Could you check a few things on this drawing? It's one solid part, dimensions in mm from its lowest x, y, z. A direction names the side the tool comes from. Coordinates: 2 decimals unless noted, no trailing zeros. Loops run counter-clockwise (first coordinate to the right, second up) from the corner with the lowest first, then second, coordinate; pieces in that order, holes last. Notation, with made-up numbers: M -22.5,4.5 L 30.5,4.5 A13 ccw 30.5,18.5 Z; hole C 30,74.25 d11. An arc over 180 degrees is marked long. Answer as a JSON object with one key per item and string values. Group by question number.
Item 1: Which directions (+Z, -Z, +X, -X, +Y, -Y) give clear straight access to the entire face, cutting with the end or side of a thin tool? Please do the marked faces 1 and 2.
Item 2: Suppose I cut it at B-B (y = 38.1). Write out the boundary of the cut face in (x, z) (1 decimal).
Item 3: If I drill on line 1 (Y direction, x = 18, z = 38) (1 decimal); line 2 (X direction, y = 38, z = 23); line 3 (X direction, y = 38.1, z = 26.5), over which ranges is the centre line in solid material (lowest first)?
Item 4: I'm going to push flat-ended pins straight in: pin 1 Ø3 at (y, z) = (18, 38) entering from +X; pin 2 Ø1.5 at (x, z) = (58.5, 33.5) entering from -Y. Where does each tip first touch, or does it pass through?
Item 5: We'd pull the mould along Y, two halves only. Please class the marked faces 3, 4, 5 and 6: +Y half, -Y half, draft (parallel to the pull), parting line (faces both ways), or undercut.
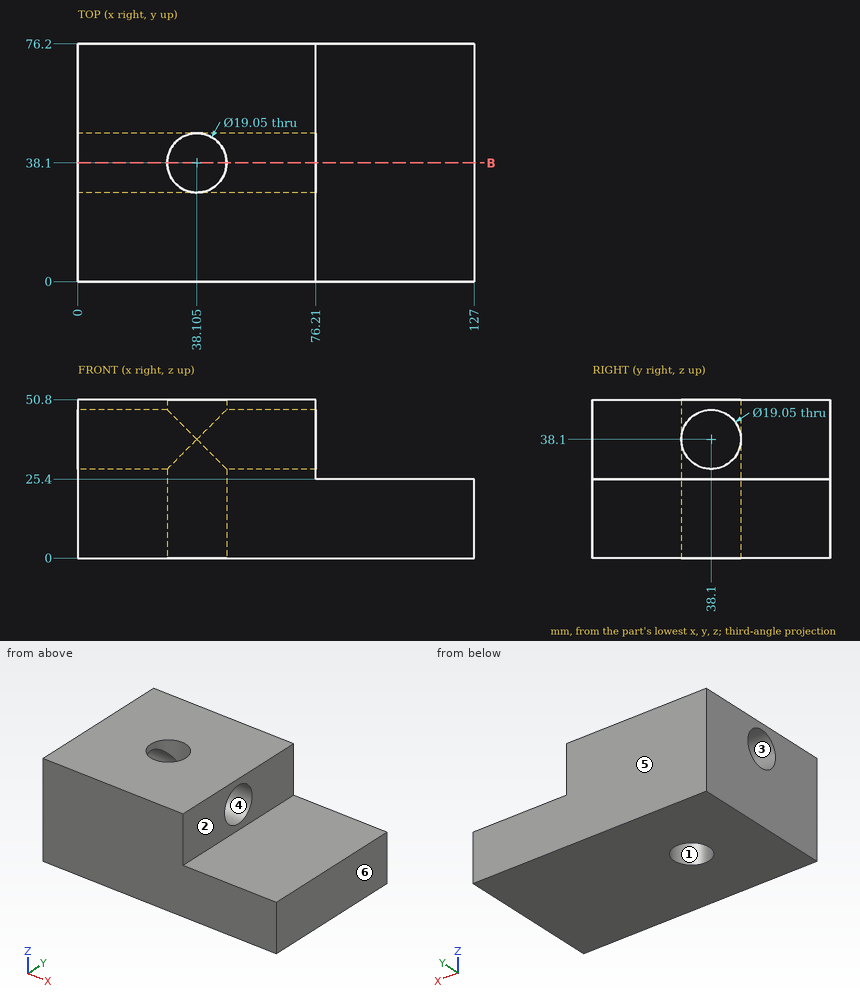
From the geometry:
{
 "1": {"face 1": "+Z, -Z", "face 2": "+Z, +X, +Y, -Y"},
 "2": {"outline": "M 0,0 L 28.6,0 L 28.6,28.6 L 0,28.6 Z; M 0,47.6 L 28.6,47.6 L 28.6,50.8 L 0,50.8 Z; M 47.6,0 L 127,0 L 127,25.4 L 76.2,25.4 L 76.2,28.6 L 47.6,28.6 Z; M 47.6,47.6 L 76.2,47.6 L 76.2,50.8 L 47.6,50.8 Z"},
 "3": {"line 1": "0 to 28.6, 47.6 to 76.2", "line 2": "0 to 28.58, 47.63 to 127", "line 3": "0 to 28.58, 47.63 to 76.21"},
 "4": {"pin 1": "x = 76.21", "pin 2": "y = 0"},
 "5": {"face 3": "undercut", "face 4": "undercut", "face 5": "+Y half", "face 6": "draft"}
}
